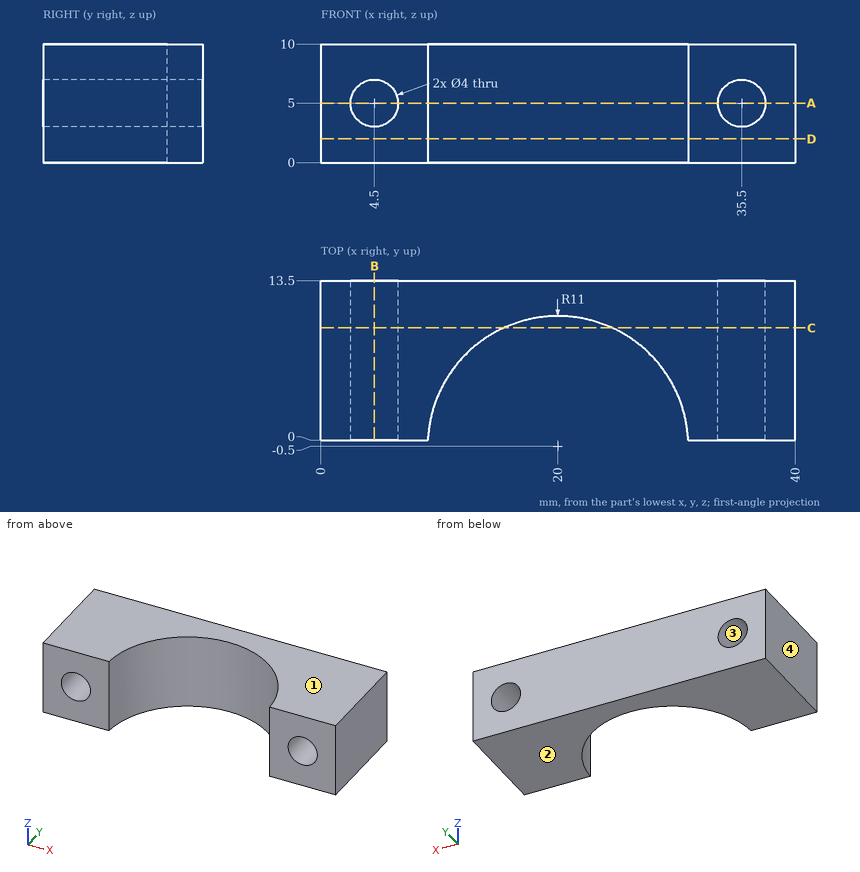
Print and shaded views of the part. All mm, measured from the part's lowest x, y and z. Round coordinates to 2 decimals unless told otherwise and drop trailing zeros. Write each loop counter-clockwise with the first axis right and the second up, starting at its lowest first coordinate (ties: lowest second). Pieces come first, ordered by that corner, then holes. Notation, with made-up numbers: (-4, 78.25) -> (52, 78.25) arc R24 ccw to (52, 103.25) -> close; hole circle Ø7 at (69, 80.25). An arc over 180 degrees is marked (long way). Return JSON: item names as keys, results as strings. Group by question number.
Q1. Mould opens along Z. For the marked faces 1, 2, 3 and 4 say: pulls with the +Z half, pulls with the -Z half, needs draft (parallel to the pull), parting line crosses it, or undercut.
Q2. Probe L1, parallel to X at y = 3, z = 5; L2, parallel to X at y = 7, z = 6.25; L3, parallel to Z at x = 35.5, y = 5.75. List the from-to ranges inside material, lowest first. Write a range as [from, to].
Q3. Saw through at C-C on y = 9.5. Write the cut outline in (x, z), plus the area to 3 significant figures.
Q4. Saw through at D-D on z = 2. Write the cut outline in (x, y).
Q5. Saw through at B-B on x = 4.5. Write the cut outline in (y, z), plus the area to 3 significant figures.
Q6. Saw through at A-A on z = 5. Write the cut outline in (x, y), plus the area to 3 significant figures.
Q7. Pin check, flat tips, straight feed: pin 1 (1.5 mm diameter, centred on x = 13, y = 4, fed in from +Z); pin 2 (3 mm diameter, centred on x = 21, z = 7, fed in from -Y). Stop position of each tip, or through.
Answer:
{
 "1": {"face 1": "pulls with the +Z half", "face 2": "pulls with the -Z half", "face 3": "undercut", "face 4": "needs draft"},
 "2": {"L1": "[0, 2.5], [6.5, 9.57], [30.43, 33.5], [37.5, 40]", "L2": "[0, 2.94], [6.06, 11.95], [28.05, 33.94], [37.06, 40]", "L3": "[0, 3], [7, 10]"},
 "3": {"outline": "(0, 0) -> (15.42, 0) -> (15.42, 10) -> (0, 10) -> close; (24.58, 0) -> (40, 0) -> (40, 10) -> (24.58, 10) -> close; hole circle Ø4 at (4.5, 5); hole circle Ø4 at (35.5, 5)", "area": "283 mm2"},
 "4": {"outline": "(0, 0) -> (9.01, 0) arc R11 cw to (30.99, 0) -> (40, 0) -> (40, 13.5) -> (0, 13.5) -> close"},
 "5": {"outline": "(0, 0) -> (13.5, 0) -> (13.5, 3) -> (0, 3) -> close; (0, 7) -> (13.5, 7) -> (13.5, 10) -> (0, 10) -> close", "area": "81.0 mm2"},
 "6": {"outline": "(0, 0) -> (2.5, 0) -> (2.5, 13.5) -> (0, 13.5) -> close; (6.5, 0) -> (9.01, 0) arc R11 cw to (30.99, 0) -> (33.5, 0) -> (33.5, 13.5) -> (6.5, 13.5) -> close; (37.5, 0) -> (40, 0) -> (40, 13.5) -> (37.5, 13.5) -> close", "area": "253 mm2"},
 "7": {"pin 1": "through", "pin 2": "y = 10.21"}
}
